```python
from build123d import *

# Parameters (mm, degrees)
MAIN_BODY_DEPTH                    = 6.35
POCKET_OUTER_SURFACE_DEPTH         = 43.18
POCKET_INSIDE_DEPTH                = 44.45
SKETCH8_W                          = 10.16
SKETCH8_H                          = 25.4
BOTTOM_SCREW_MOUNT_DEPTH           = 10.16
BOTTOM_SCREW_MOUNT_EXTRUSION_DEPTH = 10.16
LIGHT_SOCKETS_DEPTH                = 184.078329957
LIGHT_SOCKETS_DEPTH_BACK           = 6.35
SKETCH17_R                         = 4.064
SKETCH18_R                         = 9.144
LIGHT_LIP_LINERS_DEPTH             = 2.54
LIGHT_LIP_SOCKETS_REACH            = 185.078
SKETCH17_2_R                       = 4.064
TAB_SLOTS_DEPTH                    = 1.778


# Sheet-metal steps are written as plain solids
with BuildPart() as part:
    # Sketch1 → Main Body (new body)
    with BuildSketch(Plane.XY):
        Polygon((-53.975, 0), (53.975, 0), (57.15, 82.161327118), (101.6, 101.6), (101.6, 146.05), (-101.6, 146.05), (-101.6, 101.6), (-57.15, 82.161327118), align=None)
    extrude(amount=-MAIN_BODY_DEPTH)

    # Sketch6 → Pocket-Outer Surface (add)
    with BuildSketch(Plane.XY):
        Polygon((53.975, 0), (-53.975, 0), (-57.15, 82.161327118), (57.15, 82.161327118), align=None)
    extrude(amount=POCKET_OUTER_SURFACE_DEPTH)

    # Sketch7 → Pocket-Inside (cut)
    with BuildSketch(Plane(origin=(0, 0, -6.35), x_dir=(-1, 0, 0), z_dir=(0, 0, -1))):
        Polygon((-50.564894027, 76.2), (-47.86564661, 6.35), (47.86564661, 6.35), (50.564894027, 76.2), align=None)
    extrude(amount=-POCKET_INSIDE_DEPTH, mode=Mode.SUBTRACT)

    # Sketch8 → Bottom Screw Mount (add)
    with BuildSketch(Plane.XZ):
        with Locations((-48.895, 6.35)):
            Rectangle(SKETCH8_W, SKETCH8_H)
    bottom_screw_mount = extrude(amount=BOTTOM_SCREW_MOUNT_DEPTH)

    # Sketch9 → Bottom Screw Mount Extrusion (cut)
    with BuildSketch(Plane.ZY.offset(53.975)):
        Polygon((-3.81, -10.16), (19.05, -10.16), (19.05, 0), align=None)
    bottom_screw_mount_extrusion = extrude(amount=-BOTTOM_SCREW_MOUNT_EXTRUSION_DEPTH, mode=Mode.SUBTRACT)

    # Left Bottom Screw Mount: Bottom Screw Mount, Bottom Screw Mount Extrusion across plane
    add(bottom_screw_mount.mirror(Plane(origin=(0, 0, 0), x_dir=(0, 0, 1), z_dir=(1, 0, 0))))
    add(bottom_screw_mount_extrusion.mirror(Plane(origin=(0, 0, 0), x_dir=(0, 0, 1), z_dir=(1, 0, 0))), mode=Mode.SUBTRACT)

    # Sketch17 → Light Sockets (cut, two sides: drawn at the far end of the back side and taken through both)
    with BuildSketch(Plane.XY.offset(-LIGHT_SOCKETS_DEPTH_BACK)):
        with Locations((85.852, 123.825)):
            Circle(SKETCH17_R)
        with Locations((-85.852, 123.825)):
            Circle(SKETCH17_R)
        with BuildLine():
            Line((-5.969, 131.318), (5.969, 131.318))
            ThreePointArc((5.969, 131.318), (13.462, 123.825), (5.969, 116.332))
            Line((5.969, 116.332), (-5.969, 116.332))
            ThreePointArc((-5.969, 116.332), (-13.462, 123.825), (-5.969, 131.318))
        make_face()
    extrude(amount=LIGHT_SOCKETS_DEPTH + LIGHT_SOCKETS_DEPTH_BACK, mode=Mode.SUBTRACT)

    # Sketch18 → Light Lip Liners (add)
    with BuildSketch(Plane.XY):
        with Locations((-85.852, 123.825)):
            Circle(SKETCH18_R)
        with Locations((85.852, 123.825)):
            Circle(SKETCH18_R)
        with BuildLine():
            Line((5.969, 136.398), (-5.969, 136.398))
            ThreePointArc((-5.969, 136.398), (-18.542, 123.825), (-5.969, 111.252))
            Line((-5.969, 111.252), (5.969, 111.252))
            ThreePointArc((5.969, 111.252), (18.542, 123.825), (5.969, 136.398))
        make_face()
    extrude(amount=LIGHT_LIP_LINERS_DEPTH)

    # Sketch17<2> → Light Lip Sockets (cut, up to next)
    with BuildSketch(Plane.XY, mode=Mode.PRIVATE) as light_lip_sockets_sk1:
        with Locations((85.852, 123.825)):
            Circle(SKETCH17_2_R)
    light_lip_sockets_tool1 = extrude(light_lip_sockets_sk1.sketch, amount=LIGHT_LIP_SOCKETS_REACH, mode=Mode.PRIVATE) & part.part
    # Sketch17<2> → Light Lip Sockets (cut, up to next)
    with BuildSketch(Plane.XY, mode=Mode.PRIVATE) as light_lip_sockets_sk2:
        with Locations((-85.852, 123.825)):
            Circle(SKETCH17_2_R)
    light_lip_sockets_tool2 = extrude(light_lip_sockets_sk2.sketch, amount=LIGHT_LIP_SOCKETS_REACH, mode=Mode.PRIVATE) & part.part
    # Sketch17<2> → Light Lip Sockets (cut, up to next)
    with BuildSketch(Plane.XY, mode=Mode.PRIVATE) as light_lip_sockets_sk3:
        with BuildLine():
            Line((-5.969, 131.318), (5.969, 131.318))
            ThreePointArc((5.969, 131.318), (13.462, 123.825), (5.969, 116.332))
            Line((5.969, 116.332), (-5.969, 116.332))
            ThreePointArc((-5.969, 116.332), (-13.462, 123.825), (-5.969, 131.318))
        make_face()
    light_lip_sockets_tool3 = extrude(light_lip_sockets_sk3.sketch, amount=LIGHT_LIP_SOCKETS_REACH, mode=Mode.PRIVATE) & part.part
    add(light_lip_sockets_tool1.solids().sort_by_distance((85.852, 123.825, 0))[0], mode=Mode.SUBTRACT)
    add(light_lip_sockets_tool2.solids().sort_by_distance((-85.852, 123.825, 0))[0], mode=Mode.SUBTRACT)
    add(light_lip_sockets_tool3.solids().sort_by_distance((0, 123.825, 0))[0], mode=Mode.SUBTRACT)

    # Sketch19 → Tab Slots (cut)
    with BuildSketch(Plane(origin=(0, 0, -6.35), x_dir=(-1, 0, 0), z_dir=(0, 0, -1))):
        with BuildLine():
            Line((72.263, 146.05), (72.263, 123.825))
            ThreePointArc((72.263, 123.825), (85.852, 110.236), (99.441, 123.825))
            Line((99.441, 123.825), (99.441, 146.05))
            Line((99.441, 146.05), (72.263, 146.05))
        make_face()
    tab_slots = extrude(amount=-TAB_SLOTS_DEPTH, mode=Mode.SUBTRACT)

    # Mirror3: Tab Slots across plane
    add(tab_slots.mirror(Plane(origin=(0, 0, 0), x_dir=(0, 0, 1), z_dir=(1, 0, 0))), mode=Mode.SUBTRACT)


solid = part.part
```
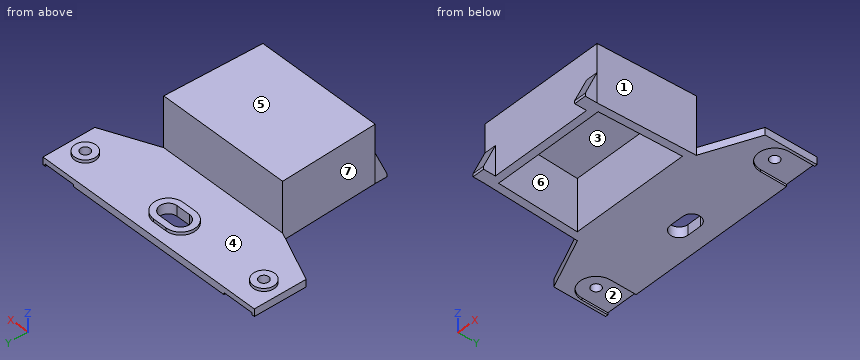
Here's how the part is built. I have some questions about the finished solid (model axes, mm). Face numbers are marked on the shaded views. A direction names the side the tool comes from. Coordinates: 2 decimals unless noted, no trailing zeros. Order: outer loops, then holes, each group sorted by start corner. A loop starts at its lowest first (then second) coordinate and runs counter-clockwise, first axis right, second up. Notation, with made-up numbers: (-35, 44.25) -> (24, 44.25) arc R17 cw to (24, 77.25) -> close; hole circle Ø5 at (1, 15.25). An arc over 180 degrees is marked (long way). Return JSON: item names as keys, results as strings.
1) Thinking about a two-plate mould opening in X: for the marked faces 5, 6 and 7, which applies, +X half, -X half, draft (parallel to the pull), parting line (faces both ways), or undercut?
Conclusion:
{"face 5": "draft", "face 6": "undercut", "face 7": "-X half"}
2) If we section it at D-D on z = 8.5: List the corners of the cut face in (x, y) for me (3 decimals), plus the area to 3 significant figures.
Conclusion:
{"outline": "(-57.15, 82.161) -> (-53.975, 0) -> (-53.975, -4.689) -> (-43.815, -4.689) -> (-43.815, 0) -> (43.815, 0) -> (43.815, -4.689) -> (53.975, -4.689) -> (53.975, 0) -> (57.15, 82.161) -> close; hole (-50.565, 76.2) -> (-47.866, 6.35) -> (47.866, 6.35) -> (50.565, 76.2) -> close", "area": "2,350 mm²"}
3) If I drill on probe 1 along X at (y, z) = (116, 2); probe 2 along Y at (x, z) = (-28, 2); probe 3 along Z at (x, y) = (-36, 20), over which ranges is the centre line in solid material (lowest first)?
Conclusion:
{"probe 1": "x = -90.58 to -81.12, -15.81 to 15.81, 81.12 to 90.58", "probe 2": "y = 0 to 6.35, 76.2 to 82.16", "probe 3": "z = 38.1 to 43.18"}
4) On a 3-axis mill with a long thin cutter (end or side, diameter ignored), from which of +Z, -Z, +X, -X, +Y, -Y can I reach the whole of each face in a straight line? I mean the marked faces 1, 2, 3 and 4. Say none if no direction works.
Conclusion:
{"face 1": "+Z, -Z, +X, -Y", "face 2": "-Z, +Y", "face 3": "-Z", "face 4": "+Z"}
5) If we section it at C-C on y = 21.5: List the corners of the cut face in (x, z) for me.
Conclusion:
{"outline": "(-54.81, -6.35) -> (-48.45, -6.35) -> (-48.45, 38.1) -> (48.45, 38.1) -> (48.45, -6.35) -> (54.81, -6.35) -> (54.81, 43.18) -> (-54.81, 43.18) -> close"}
6) If we section it at A-A on z = 23: List the corners of the cut face in (x, y) for me (3 decimals).
Conclusion:
{"outline": "(-57.15, 82.161) -> (-53.975, 0) -> (53.975, 0) -> (57.15, 82.161) -> close; hole (-50.565, 76.2) -> (-47.866, 6.35) -> (47.866, 6.35) -> (50.565, 76.2) -> close"}
7) I'm going to push flat-ended pins straight in: P1, Ø13.5, axis at x = 24, z = 12, coming from the -Y side; P2, Ø8, axis at x = 3.5, z = 5, coming from the +Y side; P3, Ø5.5, axis at x = 85, y = 121.5, coming from the +Z side. Where does each tip first touch, or does it pass through?
Conclusion:
{"P1": "stops at y = 0", "P2": "stops at y = 136.4", "P3": "stops at z = 2.54"}
8) If we section it at B-B on x = 32: List the corners of the cut face in (y, z) for me.
Conclusion:
{"outline": "(0, -6.35) -> (6.35, -6.35) -> (6.35, 38.1) -> (76.2, 38.1) -> (76.2, -6.35) -> (146.05, -6.35) -> (146.05, 0) -> (82.16, 0) -> (82.16, 43.18) -> (0, 43.18) -> close"}
